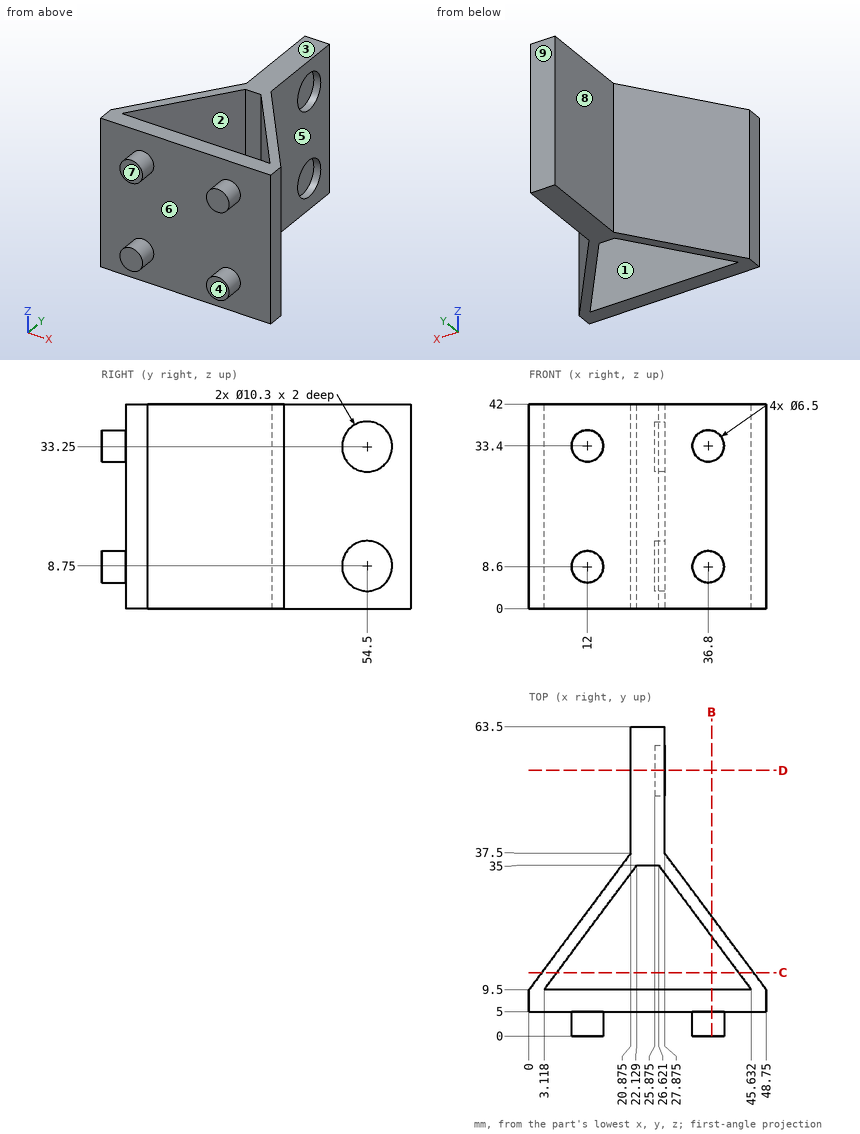
Answer from the drawing. Dimensions are ordinates in mm from the lowest x, y and z of the part. A direction names the side the tool comes from. Coordinates: 2 decimals unless noted, no trailing zeros. Loops run counter-clockwise (first coordinate to the right, second up) from the corner with the lowest first, then second, coordinate; pieces in that order, holes last. Notation, with made-up numbers: (-20, 55.5) - (38, 55.5) arc R13 ccw to (38, 69.5) - close; hole circle Ø9 at (20.5, -35). An arc over 180 degrees is marked (long way). Answer in a Markdown table with one row per item.
1. Which of the six approach directions +Z, -Z, +X, -X, +Y, -Y give full straight-line access (tool end or side, diameter ignored) to the marked faces 5, 6, 7, 8 and 9?
Conclusion:
| item | result |
|---|---|
| face 5 | +Z, -Z, +X, +Y |
| face 6 | -Y |
| face 7 | +Z, -Z, +X, -X, -Y |
| face 8 | +Z, -Z, -X, +Y |
| face 9 | +Z, -Z, +X, -X, +Y |
2. Given pin 1 (5 mm diameter, centred on x = 24, z = 21.5, fed in from -Y); pin 2 (2 mm diameter, centred on y = 18, z = 34, fed in from +X); pin 3 (13 mm diameter, centred on y = 53, z = 28.5, fed in from +X) (3 decimals), each flat-ended and moving along its own axis, determine where each tip first touches the part or whether it passes through.
Conclusion:
| item | result |
|---|---|
| pin 1 | stops at y = 5 |
| pin 2 | stops at x = 43.16 |
| pin 3 | stops at x = 27.875 |
3. Straight lines are drawn through the part: line 1 (Z direction, x = 27, y = 54) (1 decimal); line 2 (Y direction, x = 26.5, z = 33.25); line 3 (Y direction, x = 24.5, z = 30). For each, find the intervals that lie inside material, in ascending order.
Conclusion:
| item | result |
|---|---|
| line 1 | z = 0 to 3.6, 13.9 to 28.1, 38.4 to 42 |
| line 2 | y = 5 to 9.5, 35 to 49.35, 59.65 to 63.5 |
| line 3 | y = 5 to 9.5, 35 to 63.5 |
4. Find section B-B, the plane x = 37.5. Write down the section's boundary in (y, z).
Conclusion:
| item | result |
|---|---|
| outline | (0, 5.43) - (5, 5.43) - (5, 0) - (9.5, 0) - (9.5, 42) - (5, 42) - (5, 36.57) - (0, 36.57) - (0, 30.23) - (5, 30.23) - (5, 11.77) - (0, 11.77) - close; (20.41, 0) - (24.59, 0) - (24.59, 42) - (20.41, 42) - close |
5. Find section D-D, the plane y = 54.5. Write down the section's boundary in (x, z) (1 decimal), then the cut area to 3 significant figures.
Conclusion:
| item | result |
|---|---|
| outline | (20.9, 0) - (27.9, 0) - (27.9, 3.6) - (25.9, 3.6) - (25.9, 13.9) - (27.9, 13.9) - (27.9, 28.1) - (25.9, 28.1) - (25.9, 38.4) - (27.9, 38.4) - (27.9, 42) - (20.9, 42) - close |
| area | 253 mm² |
6. Find section C-C, the plane y = 13. Write down the section's boundary in (x, z).
Conclusion:
| item | result |
|---|---|
| outline | (2.61, 0) - (5.73, 0) - (5.73, 42) - (2.61, 42) - close; (43.02, 0) - (46.14, 0) - (46.14, 42) - (43.02, 42) - close |
7. Determine the mould class of the marked faces 1, 2, 3 and 4 for opening direction Y: +Y half, -Y half, draft (parallel to the pull), parting line (faces both ways), or undercut.
Conclusion:
| item | result |
|---|---|
| face 1 | undercut |
| face 2 | undercut |
| face 3 | draft |
| face 4 | -Y half |
